The model under review builds one solid part; all positions refer to its coordinate system, in mm. A direction names the side the tool comes from. Round coordinates to 2 decimals unless told otherwise and drop trailing zeros. Loops run counter-clockwise (first coordinate to the right, second up) from the corner with the lowest first, then second, coordinate; pieces in that order, holes last. Notation, with made-up numbers: M 76,64 L 111,64 A15 ccw 111,69 Z; hole C 43.25,-17.75 d6. An arc over 180 degrees is marked long. Return JSON: item names as keys, results as strings. Group by question number.
Q1. For faces 4 (the face through (27, 49, 8)), 5 (the face through (42, 49, 13.5)), 6 (the face through (49.044, 50.001, 12.385)), list the 3-axis set-ups (+Z, -Z, +X, -X, +Y, -Y) from which the entire face can be reached by the end or side of a thin tool; tool diameter is ignored.
Q2. Consider section B-B (z = 15.25). State the section outline as (x, y) points, and give its area (3 significant figures).
Q3. Clearance check with flat-ended pins moving along their axes: pin 1 Ø5.5 at (y, z) = (48.5, 9) entering from +X; pin 2 Ø8 at (x, y) = (41.5, 31.5) entering from -Z; pin 3 Ø5 at (y, z) = (47.5, 5) entering from +X; pin 4 Ø12 at (y, z) = (27, 8) entering from +X. State where each tip first meets the part, or that it passes through.
Q4. Consider section C-C (y = 77). State the section outline as (x, z) points.
Q5. Draft analysis for pull direction X (two halves, no side actions). For faces 1 (the face through (44, 49, 12)), 2 (the face through (-12, 50, 0)), 3 (the face through (47, 49, 12)), state which applies: pulls with the +X half, pulls with the -X half, needs draft (parallel to the pull), parting line crosses it, or undercut.
Q6. Consider section D-D (x = 35). State the section outline as (y, z) points, and give its area (3 significant figures).
Q7. To check wall thickness, follow line 1 along X through (y, z) = (49.5, 18.25); line 2 along Z through (x, y) = (27.95, 49.25); line 3 along Y through (x, z) = (2.25, 10). State the ranges of each line that lie inside material, in increasing order.
Q8. Consider section A-A (x = 15). State the section outline as (y, z) points, and give its area (4 significant figures).
from build123d import *

# Parameters (mm, degrees)
SKETCH_1_W          = 18
SKETCH_1_H          = 63.5
SKETCH_1_R          = 5
EXTRUDE_1_DEPTH     = 17
EXTRUDE_1_2_DEPTH   = 17
SKETCH_2_W          = 60
SKETCH_2_H          = 63.5
SKETCH_2_R          = 5
SKETCH_2_R_2        = 12
EXTRUDE_2_DEPTH     = 3
SKETCH_3_W          = 3
SKETCH_3_H          = 63.5
EXTRUDE_3_DEPTH     = 10
RIB_1_REACH         = 88.355
SKETCH_4_WALL_W     = 194.433823758
SKETCH_4_WALL_H     = 63.5
SKETCH_7_W          = 3
SKETCH_7_H          = 7
CUT_EXTRUDE_1_DEPTH = 3.5
HOLE_WIZARD_1_D     = 3.2
SKETCH_13_R         = 2.5
CUT_EXTRUDE_2_DEPTH = 11
SKETCH_14_W         = 2
SKETCH_14_H         = 35
CUT_EXTRUDE_3_DEPTH = 1


with BuildPart() as part:
    # Sketch 1 → Extrude 1 (new body)
    with BuildSketch(Plane.XY):
        with Locations((36, 49.25)):
            Rectangle(SKETCH_1_W, SKETCH_1_H)
        with Locations((35, 49.25)):
            Circle(SKETCH_1_R, mode=Mode.SUBTRACT)
    extrude(amount=EXTRUDE_1_DEPTH)



with BuildPart() as body_2:
    # Sketch 1 → Extrude 1 2 (new body)
    with BuildSketch(Plane.XY):
        with Locations((-6, 49.25)):
            Rectangle(SKETCH_1_W, SKETCH_1_H)
        with Locations((-5, 49.25)):
            Circle(SKETCH_1_R, mode=Mode.SUBTRACT)
    extrude(amount=EXTRUDE_1_2_DEPTH)


with BuildPart() as part_1:
    add(part.part)

    add(body_2.part)  # Extrude 2 merges body 2
    # Sketch 2 → Extrude 2 (add)
    with BuildSketch(Plane.XY.offset(17)):
        with Locations((15, 49.25)):
            Rectangle(SKETCH_2_W, SKETCH_2_H)
        with Locations((35, 49.25)):
            Circle(SKETCH_2_R, mode=Mode.SUBTRACT)
        with Locations((-5, 49.25)):
            Circle(SKETCH_2_R, mode=Mode.SUBTRACT)
        with Locations((15, 49.25)):
            Circle(SKETCH_2_R_2, mode=Mode.SUBTRACT)
    extrude(amount=EXTRUDE_2_DEPTH)

    # Sketch 3 → Extrude 3 (add)
    with BuildSketch(Plane(origin=(45, 0, 0), x_dir=(0, 0, -1), z_dir=(1, 0, 0))):
        with Locations((-18.5, 49.25)):
            Rectangle(SKETCH_3_W, SKETCH_3_H)
    extrude(amount=EXTRUDE_3_DEPTH)

    # Sketch 4 wall → Rib 1 (add, up to next)
    with BuildSketch(Plane(origin=(50, 17.5, 8.5), x_dir=(-0.507020126563, 0, -0.861934215158), z_dir=(0.861934215158, 0, -0.507020126563)), mode=Mode.PRIVATE) as rib_1_sk1:
        with Locations((0, 31.75)):
            Rectangle(SKETCH_4_WALL_W, SKETCH_4_WALL_H)
    rib_1_tool1 = extrude(rib_1_sk1.sketch, amount=-RIB_1_REACH, mode=Mode.PRIVATE) - part_1.part
    add(rib_1_tool1.solids().sort_by_distance((50, 17.5, 8.5))[0])

    # Sketch 7 → Cut-Extrude 1 (cut, symmetric)
    with BuildSketch(Plane.XY.offset(10)):
        with Locations((-12.5, 49.25)):
            Rectangle(SKETCH_7_W, SKETCH_7_H)
        with Locations((42.5, 49.25)):
            Rectangle(SKETCH_7_W, SKETCH_7_H)
    extrude(amount=CUT_EXTRUDE_1_DEPTH, both=True, mode=Mode.SUBTRACT)

    # Hole Wizard 1 (through all)
    with Locations(Plane.ZY.offset(15)):
        with Locations((10, 49.25)):
            Hole(HOLE_WIZARD_1_D / 2)

    # Sketch 13 → Cut-Extrude 2 (cut)
    with BuildSketch(Plane.ZY.offset(-47)):
        with Locations((10, 49.25)):
            Circle(SKETCH_13_R)
    extrude(amount=-CUT_EXTRUDE_2_DEPTH, mode=Mode.SUBTRACT)

    # Sketch 14 → Cut-Extrude 3 (cut)
    with BuildSketch(Plane.ZY.offset(15)):
        with Locations((0, 49.25)):
            Rectangle(SKETCH_14_W, SKETCH_14_H)
    extrude(amount=-CUT_EXTRUDE_3_DEPTH, mode=Mode.SUBTRACT)


solid = part_1.part
Values:
{
 "1": {"face 4": "-Z, +Y, -Y", "face 5": "none", "face 6": "+X"},
 "2": {"outline": "M -15,17.5 L 3,17.5 L 3,81 L -15,81 Z; M 27,17.5 L 53.97,17.5 L 53.97,81 L 27,81 Z; hole C -5,49.25 d10; hole C 35,49.25 d10", "area": "2,700 mm2"},
 "3": {"pin 1": "stops at x = 51.72", "pin 2": "stops at z = 0", "pin 3": "stops at x = 49.41", "pin 4": "stops at x = 53.24"},
 "4": {"outline": "M -15,0 L 3,0 L 3,17 L 27,17 L 27,0 L 45,0 L 55,17 L 55,20 L -15,20 Z"},
 "5": {"face 1": "undercut", "face 2": "needs draft", "face 3": "pulls with the +X half"},
 "6": {"outline": "M 17.5,0 L 44.25,0 L 44.25,20 L 17.5,20 Z; M 54.25,0 L 81,0 L 81,20 L 54.25,20 Z", "area": "1,070 mm2"},
 "7": {"line 1": "x = -15 to -9.99, -0.01 to 3, 27 to 30.01, 39.99 to 55", "line 2": "z = 0 to 8.4, 11.6 to 20", "line 3": "y = 17.5 to 47.65, 50.85 to 81"},
 "8": {"outline": "M 17.5,17 L 37.25,17 L 37.25,20 L 17.5,20 Z; M 61.25,17 L 81,17 L 81,20 L 61.25,20 Z", "area": "118.5 mm2"}
}
